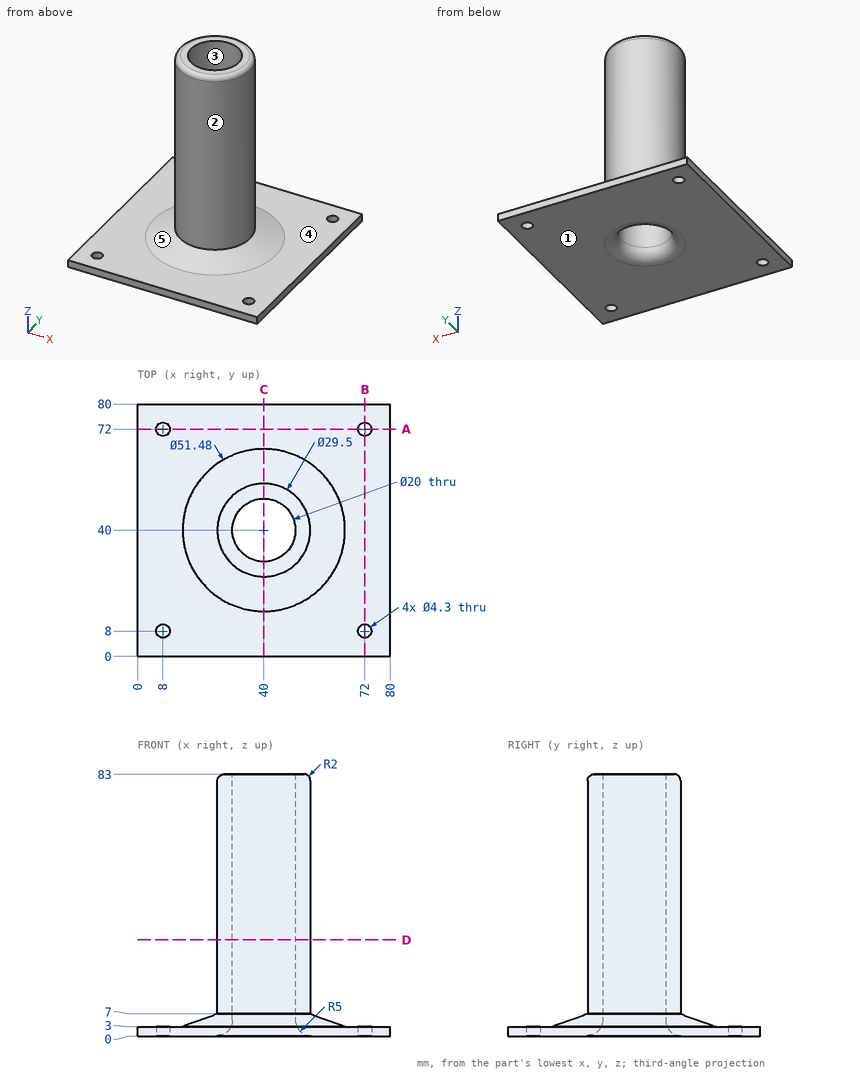
Part print with two shaded views. Sizes in mm from the minimum x, y, z corner. A direction names the side the tool comes from. Coordinates: 2 decimals unless noted, no trailing zeros. Order: outer loops, then holes, each group sorted by start corner. A loop starts at its lowest first (then second) coordinate and runs counter-clockwise, first axis right, second up. Notation, with made-up numbers: (-9.75, -39) - (41.25, -39) arc R33 ccw to (41.25, -5) - close; hole circle Ø11 at (22, -22.5). An arc over 180 degrees is marked (long way). Write item = value, one per line. Start each with the question number.
1) Saw through at C-C on x = 40. Write the cut outline in (y, z).
2) Flat gauge pins, fed straight in: pin 1 Ø1.5 at (y, z) = (35, 19) entering from -X; pin 2 Ø10 at (x, z) = (21.5, 53.5) entering from +Y; pin 3 Ø5 at (x, y) = (72, 8) entering from +Z. Where does each tip first touch, or does it go through?
3) Saw through at D-D on z = 30.5. Write the cut outline in (x, y), then the cut area to 3 significant figures.
4) Two-plate mould, pull along X, no slides. Class the marked faces 3, 4 and 5: pulls with the +X half, pulls with the -X half, needs draft (parallel to the pull), parting line crosses it, or undercut.
5) 3-axis set-ups, long thin cutter, end or side, ignore diameter. For the marked faces 1 and 2: which of +Z, -Z, +X, -X, +Y, -Y reach the whole face in a straight line?
6) Saw through at A-A on y = 72. Write the cut outline in (x, z).
7) Wall check: line 1 along Y through (x, z) = (8, 1.85); line 2 along Z through (x, y) = (4.5, 45); line 3 along Y through (x, z) = (43.5, 42). Give the ranges that are in metal, low to high. Write a range as from..to.
From the geometry:
q1.outline = (0, 0) - (25, 0) arc R5 ccw to (30, 5) - (30, 83) - (27.25, 83) arc R2 ccw to (25.25, 81) - (25.25, 7) - (14.26, 3) - (0, 3) - close; (50, 5) arc R5 ccw to (55, 0) - (80, 0) - (80, 3) - (65.74, 3) - (54.75, 7) - (54.75, 81) arc R2 ccw to (52.75, 83) - (50, 83) - close
q2.pin_1 = 25.88
q2.pin_2 = 45.94
q2.pin_3 = 3
q3.outline = circle Ø29.5 at (40, 40); hole circle Ø20 at (40, 40)
q3.area = 369 mm^2
q4.face_3 = undercut
q4.face_4 = needs draft
q4.face_5 = parting line crosses it
q5.face_1 = -Z, +X, -X, +Y, -Y
q5.face_2 = +Z
q6.outline = (0, 0) - (5.85, 0) - (5.85, 3) - (0, 3) - close; (10.15, 0) - (69.85, 0) - (69.85, 3) - (10.15, 3) - close; (74.15, 0) - (80, 0) - (80, 3) - (74.15, 3) - close
q7.line_1 = 0..5.85, 10.15..69.85, 74.15..80
q7.line_2 = 0..3
q7.line_3 = 25.67..30.63, 49.37..54.33
